For this review, take the finished solid that the model builds, in its own axes (mm). A direction names the side the tool comes from. Give positions to 0.01 mm unless a question says otherwise; leave off trailing zeros. Loops run counter-clockwise (first coordinate to the right, second up) from the corner with the lowest first, then second, coordinate; pieces in that order, holes last.
```python
from build123d import *

# Parameters (mm, degrees)
BOSS_EXTRUDE1_DEPTH = 0.9
BOSS_EXTRUDE4_DEPTH = 12
BOSS_EXTRUDE5_DEPTH = 7


with BuildPart() as part:
    # Sketch1 → Boss-Extrude1 (new body)
    with BuildSketch(Plane(origin=(0, 0, 0), x_dir=(1, 0, 0), z_dir=(0, 1, 0))):
        with BuildLine():
            Line((-11.05, 0), (-11.05, 28.25))
            Line((-11.05, 28.25), (-10.25, 28.25))
            ThreePointArc((-10.25, 28.25), (-7.669060249, 29.319060249), (-6.6, 31.9))
            Line((-6.6, 31.9), (6.6, 31.9))
            ThreePointArc((6.6, 31.9), (7.669060249, 29.319060249), (10.25, 28.25))
            Line((10.25, 28.25), (11.05, 28.25))
            Line((11.05, 28.25), (11.05, 0))
            Line((11.05, 0), (8.35, 0))
            Line((8.35, 0), (5.85, 2.5))
            Line((5.85, 2.5), (5.85, 4.5))
            Line((5.85, 4.5), (-5.85, 4.5))
            Line((-5.85, 4.5), (-5.85, 2.5))
            Line((-5.85, 2.5), (-8.35, 0))
            Line((-8.35, 0), (-11.05, 0))
        make_face()
    extrude(amount=BOSS_EXTRUDE1_DEPTH)

    # Sketch4 → Boss-Extrude4 (add)
    with BuildSketch(Plane.ZY.offset(9.9)):
        with BuildLine():
            Line((-9.7, 0.9), (-9.7, 6.9))
            ThreePointArc((-9.7, 6.9), (-12.2, 9.4), (-14.7, 6.9))
            Line((-14.7, 6.9), (-14.7, 0.9))
            Line((-14.7, 0.9), (-9.7, 0.9))
        make_face()
    extrude(amount=-BOSS_EXTRUDE4_DEPTH)

    # Sketch5 → Boss-Extrude5 (add)
    with BuildSketch(Plane(origin=(0, 0.9, 0), x_dir=(1, 0, 0), z_dir=(0, 1, 0))):
        with BuildLine():
            Line((10.55, 15.181742423), (10.55, 10.818257577))
            ThreePointArc((10.55, 10.818257577), (7.15, 13), (10.55, 15.181742423))
        make_face()
    extrude(amount=BOSS_EXTRUDE5_DEPTH)


solid = part.part
```
Item 1: Tool access review of faces 1 (the flat face through (2.1, 5, -12)), 2 (the flat face through (-9.9, 5, -12)), 3 (the flat face through (7.12, 0.44, -1.23)): name each direction out of +Z, -Z, +X, -X, +Y, -Y from which nothing blocks a thin tool from reaching the whole face with its end or side.
Answer:
face 1: +Z, -Z, +Y
face 2: +Z, -Z, -X, +Y
face 3: +Z, +Y, -Y
Item 2: The part is to be moulded in two halves that separate along X. For faces 4 (the flat face through (-5.85, 0.4, -3.5)), 5 (the flat face through (10.55, 4, -13)), 6 (the flat face through (-0.1, 0.4, -31.9)), say which applies: released by +X, released by -X, zero draft, split by the parting line, or undercut.
Answer:
face 4: undercut
face 5: released by +X
face 6: zero draft
Item 3: For L1, parallel to Z at x = -1.5, y = 6; L2, parallel to Y at x = 2.5, z = -9; L3, parallel to Y at x = -4, z = -12, list the stretches that pass through material, from the lowest coordinate up.
Answer:
L1: z = -14.7 to -9.7
L2: y = 0 to 0.9
L3: y = 0 to 9.39
Item 4: Clearance check with flat-ended pins moving along their axes: pin 1 Ø1 at (x, y) = (-4.5, 4) entering from -Z; pin 2 Ø4 at (y, z) = (5, -13.5) entering from +X; pin 3 Ø0.6 at (x, y) = (10.5, 0.5) entering from -Z; pin 4 Ø11 at (x, z) = (-0.5, -14.5) entering from +Y. State where each tip first meets the part, or that it passes through.
Answer:
pin 1: stops at z = -14.7
pin 2: stops at x = 10.55
pin 3: stops at z = -28.25
pin 4: stops at y = 9.4
Item 5: Take a section at A-A on y = 4. Give the boundary of the cut face in (x, z), and give its area (3 significant figures).
Answer:
outline: (-9.9, -14.7) - (2.1, -14.7) - (2.1, -9.7) - (-9.9, -9.7) - close; (10.55, -15.18) - (10.55, -10.82) arc R2.4 ccw (long way) to start
area: 73.7 mm2
Item 6: Take a section at B-B on x = -8.75. Give the boundary of the cut face in (y, z), and give its area (3 significant figures).
Answer:
outline: (0, -28.57) - (0.9, -28.57) - (0.9, -14.7) - (6.9, -14.7) arc R2.5 ccw to (6.9, -9.7) - (0.9, -9.7) - (0.9, 0) - (0, 0) - close
area: 65.5 mm2
Item 7: Take a section at D-D on x = -3.5. Give the boundary of the cut face in (y, z).
Answer:
outline: (0, -31.9) - (0.9, -31.9) - (0.9, -14.7) - (6.9, -14.7) arc R2.5 ccw to (6.9, -9.7) - (0.9, -9.7) - (0.9, -4.5) - (0, -4.5) - close
Item 8: Take a section at C-C on z = -17. Give the boundary of the cut face in (x, y), and give its area (3 significant figures).
Answer:
outline: (-11.05, 0) - (11.05, 0) - (11.05, 0.9) - (-11.05, 0.9) - close
area: 19.9 mm2
